Check sheet for the modelled part. Datum: model origin and axes. Units: mm. Give positions to 0.01 mm unless a question says otherwise; leave off trailing zeros. Order: outer loops, then holes, each group sorted by start corner. A loop starts at its lowest first (then second) coordinate and runs counter-clockwise, first axis right, second up.
Item 1: Sectioned sample at A-A on y = 26.5. Record the boundary of the cut face in (x, z), and give its area (3 significant figures).
Item 2: Material ranges on line 1 along X through (y, z) = (20.5, 1.2); line 2 along X through (y, z) = (60, 0.15); line 3 along Y through (x, z) = (-63.5, 0.5) (3 decimals), recorded low to high.
Item 3: Gauge pin test, flat ends, axial feed: P1, Ø0.8, axis at x = -86.5, z = 0.5, coming from the +Y side; P2, Ø0.8, axis at x = -73.5, z = 1, coming from the +Y side. Record the tip position at first contact, or that the pin passes through.
Item 4: Sectioned sample at B-B on x = -31. Record the boundary of the cut face in (y, z) (3 decimals), and give its area (3 significant figures).
Item 5: Sectioned sample at C-C on z = 0.4. Count the separate pieces of the cut face and the enclosed holes in it, and give its area (3 significant figures).
from build123d import *

# Parameters (mm, degrees)
BOSS_EXTRUDE1_DEPTH = 1.6
SKETCH3_R           = 0.92075
CUT_EXTRUDE1_DEPTH  = 2.54
SKETCH4_R           = 0.3
SKETCH4_R_2         = 0.300000035
CUT_EXTRUDE2_DEPTH  = 2.54


with BuildPart() as part:
    # Sketch1 → Boss-Extrude1 (new body)
    with BuildSketch(Plane.XY):
        Polygon((-19.3675, 84.416506551), (-15.810445706, 84.416506551), (-7.127679781, 72.016231702), (-5.81703651, 72.933954), (0, 64.626364903), (0, 0), (-21.2725, 0), (-21.2725, 34.925), (-41.5925, 34.925), (-41.5925, 0), (-62.54750001, 0), (-62.54750001, 34.925), (-82.86750001, 34.925), (-82.86750001, 0), (-104.14000001, 0), (-104.14000001, 64.626364903), (-98.3229635, 72.933954), (-97.01232023, 72.016231702), (-88.329554304, 84.416506551), (-84.77250001, 84.416506551), (-84.77250001, 57.15), (-60.6425, 57.15), (-60.6425, 102.87), (-43.49750001, 102.87), (-43.49750001, 57.15), (-19.3675, 57.15), align=None)
    extrude(amount=BOSS_EXTRUDE1_DEPTH)

    # Sketch3 → Cut-Extrude1 (cut)
    with BuildSketch(Plane.XY.offset(1.6)):
        with Locations((-93.50375001, 4.789717726)):
            Circle(SKETCH3_R)
        with Locations((-90.96375001, 12.257317726)):
            Circle(SKETCH3_R)
        with Locations((-90.96375001, 57.822682274)):
            Circle(SKETCH3_R)
        with Locations((-96.04375001, 12.257317726)):
            Circle(SKETCH3_R)
        with Locations((-93.50375001, 65.290282274)):
            Circle(SKETCH3_R)
        with Locations((-96.04375001, 57.822682274)):
            Circle(SKETCH3_R)
        with Locations((-10.63625, 4.789717726)):
            Circle(SKETCH3_R)
        with Locations((-8.09625, 12.257317726)):
            Circle(SKETCH3_R)
        with Locations((-13.17625, 12.257317726)):
            Circle(SKETCH3_R)
        with Locations((-8.09625, 57.822682274)):
            Circle(SKETCH3_R)
        with Locations((-10.63625, 65.290282274)):
            Circle(SKETCH3_R)
        with Locations((-13.17625, 57.822682274)):
            Circle(SKETCH3_R)
    extrude(amount=-CUT_EXTRUDE1_DEPTH, mode=Mode.SUBTRACT)

    # Sketch4 → Cut-Extrude2 (cut)
    with BuildSketch(Plane(origin=(0, 0, 0), x_dir=(-1, 0, 0), z_dir=(0, 0, -1))):
        with Locations((46.355000005, 101.37)):
            Circle(SKETCH4_R)
        with Locations((47.625000005, 101.37)):
            Circle(SKETCH4_R)
        with Locations((48.895000005, 101.37)):
            Circle(SKETCH4_R)
        with Locations((50.165000005, 101.37)):
            Circle(SKETCH4_R)
        with Locations((51.435000005, 101.37)):
            Circle(SKETCH4_R)
        with Locations((52.705000005, 101.37)):
            Circle(SKETCH4_R)
        with Locations((53.975000005, 101.37)):
            Circle(SKETCH4_R)
        with Locations((55.245000005, 101.37)):
            Circle(SKETCH4_R)
        with Locations((56.515000005, 101.37)):
            Circle(SKETCH4_R)
        with Locations((57.785000005, 101.37)):
            Circle(SKETCH4_R)
        with Locations((88.166138487, 82.256136075)):
            Circle(SKETCH4_R_2)
        with Locations((88.894580561, 81.215812979)):
            Circle(SKETCH4_R_2)
        with Locations((89.623022635, 80.175489883)):
            Circle(SKETCH4_R_2)
        with Locations((90.351464709, 79.135166786)):
            Circle(SKETCH4_R_2)
        with Locations((91.079906783, 78.09484369)):
            Circle(SKETCH4_R_2)
        with Locations((91.808348857, 77.054520594)):
            Circle(SKETCH4_R_2)
        with Locations((92.536790932, 76.014197498)):
            Circle(SKETCH4_R_2)
        with Locations((93.265233006, 74.973874401)):
            Circle(SKETCH4_R_2)
        with Locations((93.99367508, 73.933551305)):
            Circle(SKETCH4_R_2)
        with Locations((94.722117154, 72.893228209)):
            Circle(SKETCH4_R_2)
        with Locations((9.417882856, 72.893228209)):
            Circle(SKETCH4_R_2)
        with Locations((10.14632493, 73.933551305)):
            Circle(SKETCH4_R_2)
        with Locations((10.874767005, 74.973874401)):
            Circle(SKETCH4_R_2)
        with Locations((11.603209079, 76.014197498)):
            Circle(SKETCH4_R_2)
        with Locations((12.331651153, 77.054520594)):
            Circle(SKETCH4_R_2)
        with Locations((13.060093227, 78.09484369)):
            Circle(SKETCH4_R_2)
        with Locations((13.788535301, 79.135166786)):
            Circle(SKETCH4_R_2)
        with Locations((14.516977375, 80.175489883)):
            Circle(SKETCH4_R_2)
        with Locations((15.24541945, 81.215812979)):
            Circle(SKETCH4_R_2)
        with Locations((15.973861524, 82.256136075)):
            Circle(SKETCH4_R_2)
    extrude(amount=-CUT_EXTRUDE2_DEPTH, mode=Mode.SUBTRACT)


solid = part.part
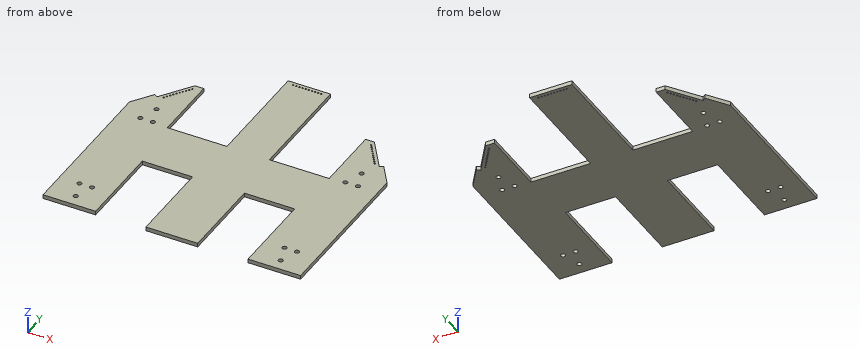
Report:
1. outline: (-104.14, 0) - (-82.87, 0) - (-82.87, 1.6) - (-104.14, 1.6) - close; (-62.55, 0) - (-41.59, 0) - (-41.59, 1.6) - (-62.55, 1.6) - close; (-21.27, 0) - (0, 0) - (0, 1.6) - (-21.27, 1.6) - close
1. area: 102 mm2
2. line 1: x = -104.14 to -82.87, -62.55 to -41.59, -21.27 to 0
2. line 2: x = -104.14 to -84.77, -60.64 to -43.5, -19.37 to 0
2. line 3: y = 34.925 to 57.15
3. P1: stops at y = 84.42
3. P2: stops at y = 57.15
4. outline: (34.925, 0) - (57.15, 0) - (57.15, 1.6) - (34.925, 1.6) - close
4. area: 35.6 mm2
5. separate pieces: 1
5. enclosed holes: 42
5. area: 6,010 mm2
